Source: CAD feature listing. Evaluate the final solid. Frame: model axes, mm. A direction names the side the tool comes from. Coordinates: 2 decimals unless noted, no trailing zeros. Order: outer loops, then holes, each group sorted by start corner. A loop starts at its lowest first (then second) coordinate and runs counter-clockwise, first axis right, second up.
Item 1: Mould query, pull axis Y, two halves, no side actions, for faces 1 (the flat face through (0, 3, 4)), 2 (the flat face through (5, 5, 4.58)), 3 (the cylindrical face through (2, 5, 5)), 4 (the flat face through (2.6, 5, 5)). Classes: released by +Y, released by -Y, zero draft, split by the parting line, or undercut.
Item 2: Ray query, line 1 (Z direction, x = 0, y = 5); line 2 (X direction, y = 4.4, z = 0.5); line 3 (Y direction, x = 5.75, z = 4.4). Return the intervals inside material, ascending.
Item 3: Contact query for flat-ended pins moving along their axis: P1, Ø0.7, axis at x = 5, z = 5, coming from the +Y side; P2, Ø1.6, axis at x = 1, y = 2, coming from the -Z side. Output: stop coordinate, or through.
Item 4: Section B-B on y = 1.85. State how many separate pieces and enclosed holes the cut face has, then the cut area to 3 significant figures.
Item 5: Section A-A on z = 5. Return the cut outline in (x, y), then the cut area to 3 significant figures.
Item 6: Reachability of faces 5 (the flat face through (6.5, 3, 0)), 6 (the flat face through (-6, 3, 0)), 7 (the flat face through (5, 5, -4.58)) from +Z, -Z, +X, -X, +Y, -Y: full face, straight path, thin tool, end or side. Return the list, or none.
Item 7: Section C-C on x = 1.5. Return the cut outline in (y, z).
from build123d import *

# Parameters (mm, degrees)
SKETCH1_W           = 13
SKETCH1_H           = 9
BOSS_EXTRUDE1_DEPTH = 6
SHELL9_START        = -6
SHELL9_OUTLINE_W    = 5.5
SHELL9_OUTLINE_H    = 8
SHELL9_DEPTH        = 12
SKETCH2_W           = 1.5
SKETCH2_H           = 4
CUT_EXTRUDE2_DEPTH  = 13.619429464
BOSS_EXTRUDE2_DEPTH = 1
CUT_EXTRUDE3_DEPTH  = 1
SKETCH6_W           = 0.84
SKETCH6_H           = 0.84
CUT_EXTRUDE4_DEPTH  = 3.9
SKETCH7_R           = 0.15
CUT_EXTRUDE6_DEPTH  = 9.9
SKETCH9_W           = 1
SKETCH9_H           = 5
CUT_EXTRUDE7_DEPTH  = 0.8


# Read off the part's stored shape, not the designer's step: Shell9
with BuildPart() as part:
    # Sketch1 → Boss-Extrude1 (new body)
    with BuildSketch(Plane(origin=(0, 0, 0), x_dir=(1, 0, 0), z_dir=(0, 1, 0))):
        Rectangle(SKETCH1_W, SKETCH1_H)
    extrude(amount=BOSS_EXTRUDE1_DEPTH)

    # Shell9 outline → Shell9 (cut)
    with BuildSketch(Plane.YZ.offset(SHELL9_START)):
        with Locations((2.75, 0)):
            Rectangle(SHELL9_OUTLINE_W, SHELL9_OUTLINE_H)
    extrude(amount=SHELL9_DEPTH, mode=Mode.SUBTRACT)

    # Sketch2 → Cut-Extrude2 (cut, through all)
    with BuildSketch(Plane.XY.offset(4.5)):
        with Locations((-1.25, 2)):
            Rectangle(SKETCH2_W, SKETCH2_H)
        with Locations((-4.25, 2)):
            Rectangle(SKETCH2_W, SKETCH2_H)
        with Locations((1.75, 2)):
            Rectangle(SKETCH2_W, SKETCH2_H)
        with Locations((4.75, 2)):
            Rectangle(SKETCH2_W, SKETCH2_H)
    extrude(amount=-CUT_EXTRUDE2_DEPTH, mode=Mode.SUBTRACT)

    # Sketch3 → Boss-Extrude2 (add)
    with BuildSketch(Plane.XY.offset(4.5)):
        with BuildLine():
            Line((2.5, 4.5), (10.5, 4.5))
            ThreePointArc((10.5, 4.5), (11, 5), (10.5, 5.5))
            Line((10.5, 5.5), (2.5, 5.5))
            ThreePointArc((2.5, 5.5), (2, 5), (2.5, 4.5))
        make_face()
    boss_extrude2 = extrude(amount=BOSS_EXTRUDE2_DEPTH)

    # Sketch5 → Cut-Extrude3 (cut)
    with BuildSketch(Plane(origin=(0, 0, 4.5), x_dir=(-1, 0, 0), z_dir=(0, 0, -1))):
        with BuildLine():
            Line((-10.5, 5.5), (-6.5, 5.5))
            Line((-6.5, 5.5), (-6.5, 4.5))
            Line((-6.5, 4.5), (-10.5, 4.5))
            ThreePointArc((-10.5, 4.5), (-11, 5), (-10.5, 5.5))
        make_face()
    cut_extrude3 = extrude(amount=-CUT_EXTRUDE3_DEPTH, mode=Mode.SUBTRACT)

    # Sketch6 → Cut-Extrude4 (cut)
    with BuildSketch(Plane(origin=(6.5, 0, 0), x_dir=(0, 0, -1), z_dir=(1, 0, 0))):
        with Locations((-5, 5)):
            Rectangle(SKETCH6_W, SKETCH6_H)
    cut_extrude4 = extrude(amount=-CUT_EXTRUDE4_DEPTH, mode=Mode.SUBTRACT)

    # Mirror1: Boss-Extrude2, Cut-Extrude3, Cut-Extrude4 across plane
    add(boss_extrude2.mirror(Plane.XY))
    add(cut_extrude3.mirror(Plane.XY), mode=Mode.SUBTRACT)
    add(cut_extrude4.mirror(Plane.XY), mode=Mode.SUBTRACT)

    # Sketch7 → Cut-Extrude6 (cut)
    with BuildSketch(Plane.XY.offset(4.58)):
        with Locations((5.75, 5.050831707)):
            Circle(SKETCH7_R)
    extrude(amount=-CUT_EXTRUDE6_DEPTH, mode=Mode.SUBTRACT)

    # Sketch9 → Cut-Extrude7 (cut)
    with BuildSketch(Plane(origin=(6.5, 0, 0), x_dir=(0, 0, -1), z_dir=(1, 0, 0))):
        with Locations((-3.3, 2.5)):
            Rectangle(SKETCH9_W, SKETCH9_H)
        with Locations((3.3, 2.5)):
            Rectangle(SKETCH9_W, SKETCH9_H)
    extrude(amount=-CUT_EXTRUDE7_DEPTH, mode=Mode.SUBTRACT)


solid = part.part
Answer list:
1. face 1: zero draft
1. face 2: undercut
1. face 3: split by the parting line
1. face 4: undercut
2. line 1: z = -4.5 to -4, 4 to 4.5
2. line 2: x = -6.5 to -6, 6 to 6.5
2. line 3: y = 0 to 4.9, 5.2 to 6
3. P1: stops at y = 5.5
3. P2: stops at z = -4.5
4. separate pieces: 10
4. enclosed holes: 0
4. area: 14.0 mm2
5. outline: (2.5, 4.5) - (6.5, 4.5) - (6.5, 4.58) - (2.6, 4.58) - (2.6, 5.42) - (6.5, 5.42) - (6.5, 5.5) - (2.5, 5.5) arc R0.5 ccw to start
5. area: 1.12 mm2
6. face 5: +Z, -Z, +X, +Y, -Y
6. face 6: -Y
6. face 7: +X
7. outline: (4, -4.5) - (6, -4.5) - (6, 4.5) - (4, 4.5) - (4, 4) - (5.5, 4) - (5.5, -4) - (4, -4) - close
